The model under review builds one solid part; all positions refer to its coordinate system, in mm. A direction names the side the tool comes from. Coordinates: 2 decimals unless noted, no trailing zeros. Write each loop counter-clockwise with the first axis right and the second up, starting at its lowest first coordinate (ties: lowest second). Pieces come first, ordered by that corner, then holes. Notation, with made-up numbers: (44, 31.25) - (53, 31.25) arc R21 ccw to (53, 65.25) - close; hole circle Ø7 at (-4, -3.5). An arc over 180 degrees is marked (long way). Use one line per item in the form item = value. Start each with the question number.
```python
from build123d import *

# Parameters (mm, degrees)
SZKIC1_W                    = 4.44
SZKIC1_H                    = 33.58
DODANIE_WYCI_GNI_CIE1_DEPTH = 1
DODANIE_WYCI_GNI_CIE2_DEPTH = 4
SZKIC3_R                    = 0.5
DODANIE_WYCI_GNI_CIE3_DEPTH = 31.58
SZKIC4_W                    = 1
SZKIC4_H                    = 0.25
WYTNIJ_WYCI_GNI_CIE1_DEPTH  = 31.58
SZKIC5_W                    = 1
SZKIC5_H                    = 0.25
WYTNIJ_WYCI_GNI_CIE2_DEPTH  = 1
SZKIC6_W                    = 4.44
SZKIC6_H                    = 1
DODANIE_WYCI_GNI_CIE5_DEPTH = 5.5
SZKIC8_R                    = 2
WYTNIJ_WYCI_GNI_CIE3_DEPTH  = 5.5
SZKIC9_W                    = 4.44
SZKIC9_H                    = 1
DODANIE_WYCI_GNI_CIE6_DEPTH = 5.5
SZKIC11_R                   = 2
WYTNIJ_WYCI_GNI_CIE4_DEPTH  = 5.5


with BuildPart() as part:
    # Szkic1 → Dodanie-wyciągnięcie1 (new body)
    with BuildSketch(Plane(origin=(0, 0, 0), x_dir=(1, 0, 0), z_dir=(0, 1, 0))):
        Rectangle(SZKIC1_W, SZKIC1_H)
    extrude(amount=DODANIE_WYCI_GNI_CIE1_DEPTH)

    # Szkic2 → Dodanie-wyciągnięcie2 (add)
    with BuildSketch(Plane(origin=(0, 1, 0), x_dir=(1, 0, 0), z_dir=(0, 1, 0))):
        Polygon((-2.22, 16.79), (-2.22, -16.79), (-1.22, -16.79), (-1.22, 15.79), (1.22, 15.79), (1.22, -16.79), (2.22, -16.79), (2.22, 16.79), align=None)
    extrude(amount=DODANIE_WYCI_GNI_CIE2_DEPTH)

    # Szkic3 → Dodanie-wyciągnięcie3 (add)
    with BuildSketch(Plane.XY.offset(-15.79)):
        with Locations(Location((0, 2.2, 0), (0, 0, 180))):
            Circle(SZKIC3_R)
    extrude(amount=DODANIE_WYCI_GNI_CIE3_DEPTH)

    # Szkic4 → Wytnij-wyciągnięcie1 (cut)
    with BuildSketch(Plane(origin=(0, 1, 0), x_dir=(1, 0, 0), z_dir=(0, 1, 0))):
        with Locations((0, -16.283529096)):
            Rectangle(SZKIC4_W, SZKIC4_H)
    extrude(amount=-WYTNIJ_WYCI_GNI_CIE1_DEPTH, mode=Mode.SUBTRACT)

    # Szkic5 → Wytnij-wyciągnięcie2 (cut)
    with BuildSketch(Plane(origin=(0, 5, 0), x_dir=(1, 0, 0), z_dir=(0, 1, 0))):
        with Locations((0, 16.29)):
            Rectangle(SZKIC5_W, SZKIC5_H)
    extrude(amount=-WYTNIJ_WYCI_GNI_CIE2_DEPTH, mode=Mode.SUBTRACT)

    # Szkic6 → Dodanie-wyciągnięcie5 (add)
    with BuildSketch(Plane.XY.offset(16.79)):
        with Locations((0, 0.5)):
            Rectangle(SZKIC6_W, SZKIC6_H)
    extrude(amount=DODANIE_WYCI_GNI_CIE5_DEPTH)

    # Szkic8 → Wytnij-wyciągnięcie3 (cut)
    with BuildSketch(Plane(origin=(0, 1, 0), x_dir=(1, 0, 0), z_dir=(0, 1, 0))):
        with Locations(Location((0, -19.539171246, 0), (0, 0, 270))):
            Circle(SZKIC8_R)
    extrude(amount=-WYTNIJ_WYCI_GNI_CIE3_DEPTH, mode=Mode.SUBTRACT)

    # Szkic9 → Dodanie-wyciągnięcie6 (add)
    with BuildSketch(Plane(origin=(0, 0, -16.79), x_dir=(-1, 0, 0), z_dir=(0, 0, -1))):
        with Locations((0, 0.5)):
            Rectangle(SZKIC9_W, SZKIC9_H)
    extrude(amount=DODANIE_WYCI_GNI_CIE6_DEPTH)

    # Szkic11 → Wytnij-wyciągnięcie4 (cut)
    with BuildSketch(Plane(origin=(0, 1, 0), x_dir=(1, 0, 0), z_dir=(0, 1, 0))):
        with Locations(Location((0, 19.54, 0), (0, 0, 270))):
            Circle(SZKIC11_R)
    extrude(amount=-WYTNIJ_WYCI_GNI_CIE4_DEPTH, mode=Mode.SUBTRACT)


solid = part.part
```
1. For L1, parallel to X at y = 0.6, z = -19.54; L2, parallel to X at y = 1.8, z = 10; L3, parallel to Z at x = 0.4, y = 0.7, list the stretches that pass through material, from the lowest coordinate up.
2. Take a section at D-D (y = 4.6). State the section outline as (x, z) points (3 decimals).
3. Take a section at B-B (x = 0). State the section outline as (y, z) points (3 decimals), plus the area to 3 significant figures.
4. Take a section at C-C (z = -19.54). State the section outline as (x, y) points, plus the area to 3 significant figures.
5. Take a section at A-A (y = 0.55). State the section outline as (x, z) points, plus the area to 3 significant figures.
6. For P1, Ø1.2, axis at x = 0.5, y = 3.5, coming from the -Z side; P2, Ø2, axis at x = 0, y = 2.5, coming from the +Z side; P3, Ø1.1, axis at x = 2, y = 4, coming from the +Z side, all flat-tipped, find the tip position at first contact; note any pin that passes through.
7. The part is to be moulded in two halves that separate along Z. For faces 1 (the flat face through (0, 3, -16.79)), 2 (the flat face through (0, 4.5, -16.165)), 3 (the flat face through (0, 0, 0)), say which applies: released by +Z, released by -Z, zero draft, split by the parting line, or undercut.
8. For faces 4 (the flat face through (1.22, 3, 0)), 5 (the cylindrical face through (0.108, 2.688, -0.221)), 6 (the flat face through (2, 3, 16.79)), 7 (the flat face through (0, 0.5, 16.409)), list the 3-axis set-ups (+Z, -Z, +X, -X, +Y, -Y) from which the entire face can be reached by the end or side of a thin tool; tool diameter is ignored.
Returned:
q1.L1 = -2.22 to -2, 2 to 2.22
q1.L2 = -2.22 to -1.22, -0.3 to 0.3, 1.22 to 2.22
q1.L3 = -22.29 to -21.5, -17.58 to 16.16, 16.41 to 17.58, 21.5 to 22.29
q2.outline = (-2.22, -16.79) - (2.22, -16.79) - (2.22, 16.79) - (1.22, 16.79) - (1.22, -15.79) - (-1.22, -15.79) - (-1.22, 16.79) - (-2.22, 16.79) - close; hole (-0.5, -16.415) - (0.5, -16.415) - (0.5, -16.165) - (-0.5, -16.165) - close
q3.outline = (0, -22.29) - (1, -22.29) - (1, -21.54) - (0, -21.54) - close; (0, -17.54) - (1, -17.54) - (1, -16.79) - (5, -16.79) - (5, -16.415) - (4, -16.415) - (4, -16.165) - (5, -16.165) - (5, -15.79) - (2.7, -15.79) - (2.7, 15.79) - (1.7, 15.79) - (1.7, -15.79) - (1, -15.79) - (1, 16.159) - (0, 16.159) - close; (0, 16.409) - (1, 16.409) - (1, 17.539) - (0, 17.539) - close; (0, 21.539) - (1, 21.539) - (1, 22.29) - (0, 22.29) - close
q3.area = 71.7 mm²
q4.outline = (-2.22, 0) - (-2, 0) - (-2, 1) - (-2.22, 1) - close; (2, 0) - (2.22, 0) - (2.22, 1) - (2, 1) - close
q4.area = 0.440 mm²
q5.outline = (-2.22, -22.29) - (2.22, -22.29) - (2.22, 22.29) - (-2.22, 22.29) - close; hole circle Ø4 at (0, -19.54); hole circle Ø4 at (0, 19.54); hole (-0.5, 16.16) - (0.5, 16.16) - (0.5, 16.41) - (-0.5, 16.41) - close
q5.area = 173 mm²
q6.P1 = -16.79
q6.P2 = 15.79
q6.P3 = 16.79
q7.face_1 = released by -Z
q7.face_2 = undercut
q7.face_3 = zero draft
q8.face_4 = +Z, +Y
q8.face_5 = +Z
q8.face_6 = +Z, +X, -X, +Y
q8.face_7 = +Y, -Y
